Verification items for the finished model (mm, model axes). A direction names the side the tool comes from. Round coordinates to 2 decimals unless told otherwise and drop trailing zeros. Loops run counter-clockwise (first coordinate to the right, second up) from the corner with the lowest first, then second, coordinate; pieces in that order, holes last. Notation, with made-up numbers: M 78.25,55.25 L 103.25,55.25 A18 ccw 103.25,62.25 Z; hole C 7.5,41 d5. An arc over 180 degrees is marked long. Write item = value, one per line. Start each with the question number.
from build123d import *

# Parameters (mm, degrees)
F1_DEPTH = 2580


with BuildPart() as f1:
    # F0 (on Top) → F1 (new body)
    with BuildSketch(Plane.XY):
        with BuildLine():
            Line((42.968165, 45.6), (0, 45.6))
            Line((0, 45.6), (0, 43.6))
            Line((0, 43.6), (42.968165, 43.6))
            ThreePointArc((42.968165, 43.6), (49.362813, 41.658163), (53.597919, 36.488431))
            Line((53.597919, 36.488431), (64.704775, 9.585159))
            ThreePointArc((64.704775, 9.585159), (70.412961, 2.617259), (79.031835, 0))
            Line((79.031835, 0), (170.968165, 0))
            ThreePointArc((170.968165, 0), (179.587039, 2.617259), (185.295225, 9.585159))
            Line((185.295225, 9.585159), (196.402081, 36.488431))
            ThreePointArc((196.402081, 36.488431), (200.637187, 41.658163), (207.031835, 43.6))
            Line((207.031835, 43.6), (292.968165, 43.6))
            ThreePointArc((292.968165, 43.6), (299.362813, 41.658163), (303.597919, 36.488431))
            Line((303.597919, 36.488431), (314.704775, 9.585159))
            ThreePointArc((314.704775, 9.585159), (320.412961, 2.617259), (329.031835, 0))
            Line((329.031835, 0), (420.968165, 0))
            ThreePointArc((420.968165, 0), (429.587039, 2.617259), (435.295225, 9.585159))
            Line((435.295225, 9.585159), (446.402081, 36.488431))
            ThreePointArc((446.402081, 36.488431), (450.637187, 41.658163), (457.031835, 43.6))
            Line((457.031835, 43.6), (542.968165, 43.6))
            ThreePointArc((542.968165, 43.6), (549.362813, 41.658163), (553.597919, 36.488431))
            Line((553.597919, 36.488431), (564.704775, 9.585159))
            ThreePointArc((564.704775, 9.585159), (570.412961, 2.617259), (579.031835, 0))
            Line((579.031835, 0), (670.968165, 0))
            ThreePointArc((670.968165, 0), (679.587039, 2.617259), (685.295225, 9.585159))
            Line((685.295225, 9.585159), (696.402081, 36.488431))
            ThreePointArc((696.402081, 36.488431), (700.637187, 41.658163), (707.031835, 43.6))
            Line((707.031835, 43.6), (792.968165, 43.6))
            ThreePointArc((792.968165, 43.6), (799.362813, 41.658163), (803.597919, 36.488431))
            Line((803.597919, 36.488431), (814.704775, 9.585159))
            ThreePointArc((814.704775, 9.585159), (820.412961, 2.617259), (829.031835, 0))
            Line((829.031835, 0), (920.968165, 0))
            ThreePointArc((920.968165, 0), (929.587039, 2.617259), (935.295225, 9.585159))
            Line((935.295225, 9.585159), (946.402081, 36.488431))
            ThreePointArc((946.402081, 36.488431), (950.637187, 41.658163), (957.031835, 43.6))
            Line((957.031835, 43.6), (1024, 43.6))
            Line((1024, 43.6), (1024, 45.6))
            Line((1024, 45.6), (957.031835, 45.6))
            ThreePointArc((957.031835, 45.6), (949.525074, 43.320452), (944.553428, 37.251636))
            Line((944.553428, 37.251636), (933.446572, 10.348364))
            ThreePointArc((933.446572, 10.348364), (928.474926, 4.279548), (920.968165, 2))
            Line((920.968165, 2), (829.031835, 2))
            ThreePointArc((829.031835, 2), (821.525074, 4.279548), (816.553428, 10.348364))
            Line((816.553428, 10.348364), (805.446572, 37.251636))
            ThreePointArc((805.446572, 37.251636), (800.474926, 43.320452), (792.968165, 45.6))
            Line((792.968165, 45.6), (707.031835, 45.6))
            ThreePointArc((707.031835, 45.6), (699.525074, 43.320452), (694.553428, 37.251636))
            Line((694.553428, 37.251636), (683.446572, 10.348364))
            ThreePointArc((683.446572, 10.348364), (678.474926, 4.279548), (670.968165, 2))
            Line((670.968165, 2), (579.031835, 2))
            ThreePointArc((579.031835, 2), (571.525074, 4.279548), (566.553428, 10.348364))
            Line((566.553428, 10.348364), (555.446572, 37.251636))
            ThreePointArc((555.446572, 37.251636), (550.474926, 43.320452), (542.968165, 45.6))
            Line((542.968165, 45.6), (457.031835, 45.6))
            ThreePointArc((457.031835, 45.6), (449.525074, 43.320452), (444.553428, 37.251636))
            Line((444.553428, 37.251636), (433.446572, 10.348364))
            ThreePointArc((433.446572, 10.348364), (428.474926, 4.279548), (420.968165, 2))
            Line((420.968165, 2), (329.031835, 2))
            ThreePointArc((329.031835, 2), (321.525074, 4.279548), (316.553428, 10.348364))
            Line((316.553428, 10.348364), (305.446572, 37.251636))
            ThreePointArc((305.446572, 37.251636), (300.474926, 43.320452), (292.968165, 45.6))
            Line((292.968165, 45.6), (207.031835, 45.6))
            ThreePointArc((207.031835, 45.6), (199.525074, 43.320452), (194.553428, 37.251636))
            Line((194.553428, 37.251636), (183.446572, 10.348364))
            ThreePointArc((183.446572, 10.348364), (178.474926, 4.279548), (170.968165, 2))
            Line((170.968165, 2), (79.031835, 2))
            ThreePointArc((79.031835, 2), (71.525074, 4.279548), (66.553428, 10.348364))
            Line((66.553428, 10.348364), (55.446572, 37.251636))
            ThreePointArc((55.446572, 37.251636), (50.474926, 43.320452), (42.968165, 45.6))
        make_face()
    extrude(amount=F1_DEPTH)


solid = f1.part
1. Tool access check on faces 4 (the flat face through (990, 43.6, 1272)), 5 (the flat face through (749, 43.6, 1272)), 6 (the flat face through (126, 2, 1272)), 7 (the flat face through (21, 43.6, 1272)), 8 (the flat face through (501, 45.6, 1272)). Record the directions out of +Z, -Z, +X, -X, +Y, -Y that give a thin tool (end or side, any length) a straight path to the whole face; none if there is none.
2. Section check A-A, the plane x = 870. Enter the section's corners in (y, z).
3. Mould release check, pull along X, two halves, no side actions. Record for faces 1 (the flat face through (249, 43.6, 1272)), 2 (the flat face through (374, 0, 1272)), 3 (the flat face through (626, 2, 1272)): pulls with the +X half, pulls with the -X half, needs draft (parallel to the pull), parting line crosses it, or undercut.
4. Gauge pin test, flat ends, axial feed: P1, Ø3, axis at x = 716.5, z = 1841.5, coming from the -Y side; P2, Ø12, axis at y = 32.5, z = 874.5, coming from the -X side; P3, Ø1.5, axis at x = 696, z = 2065.5, coming from the -Y side. Record the tip position at first contact, or that the pin passes through.
5. Thickness scan on line 1 (Y direction, x = 966.5, z = 977.5); line 2 (Y direction, x = 401, z = 1313). Record the ranges inside material, lowest first.
Computed values:
q1.face_4 = +Z, -Z, +X, -Y
q1.face_5 = +Z, -Z, -Y
q1.face_6 = +Z, -Z, +Y
q1.face_7 = +Z, -Z, -X, -Y
q1.face_8 = +Z, -Z, +X, -X, +Y
q2.outline = M 0,0 L 2,0 L 2,2580 L 0,2580 Z
q3.face_1 = undercut
q3.face_2 = needs draft
q3.face_3 = undercut
q4.P1 = 43.6
q4.P2 = 52.52
q4.P3 = 33.7
q5.line_1 = 43.6 to 45.6
q5.line_2 = 0 to 2
